Design review of the part built by this model. Coordinates are the model's own, in mm. Face numbers are marked on the shaded views. A direction names the side the tool comes from. Give positions to 0.01 mm unless a question says otherwise; leave off trailing zeros. Loops run counter-clockwise (first coordinate to the right, second up) from the corner with the lowest first, then second, coordinate; pieces in that order, holes last. Notation, with made-up numbers: M -14,76.5 L -10,76.5 A26 cw -10,110.5 Z; hole C 26.5,-10.75 d10. An arc over 180 degrees is marked long. Use CSV: the item, a comma, the result in double quotes.
from build123d import *

# Parameters (mm, degrees)
BOSS_EXTRUDE1_DEPTH = 20.32
SKETCH2_R           = 6.858
BOSS_EXTRUDE2_DEPTH = 1.27
SKETCH3_R           = 2.9845
BOSS_EXTRUDE3_DEPTH = 4.191


with BuildPart() as part:
    # Sketch1 → Boss-Extrude1 (new body)
    with BuildSketch(Plane.XY):
        Polygon((0, 0), (40.005, 0), (40.005, 27.94), (47.117, 27.94), (47.117, 31.115), (40.005, 31.115), (40.005, 40.64), (0, 40.64), (0, 31.115), (-7.112, 31.115), (-7.112, 27.94), (0, 27.94), align=None)
    extrude(amount=BOSS_EXTRUDE1_DEPTH)

    # Sketch2 → Boss-Extrude2 (add)
    with BuildSketch(Plane(origin=(0, 40.64, 0), x_dir=(1, 0, 0), z_dir=(0, 1, 0))):
        with Locations((10.886333584, -10.16)):
            Circle(SKETCH2_R)
    extrude(amount=BOSS_EXTRUDE2_DEPTH)

    # Sketch3 → Boss-Extrude3 (add)
    with BuildSketch(Plane(origin=(0, 41.91, 0), x_dir=(1, 0, 0), z_dir=(0, 1, 0))):
        with Locations((10.886333584, -10.16)):
            Circle(SKETCH3_R)
    extrude(amount=BOSS_EXTRUDE3_DEPTH)


solid = part.part
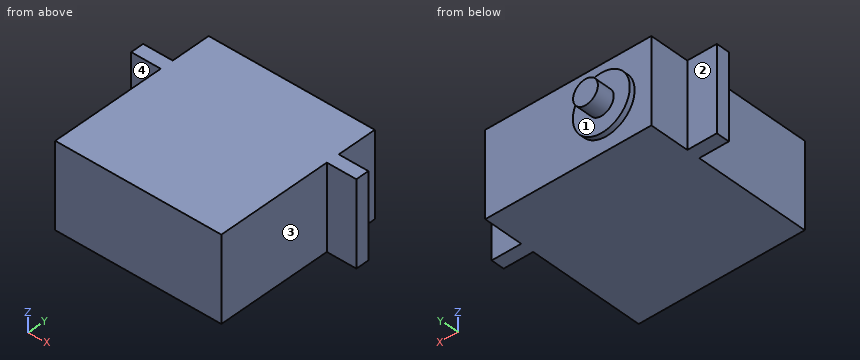
(1) We need section C-C on y = 26. State the section outline as (x, z) points (3 decimals), then the cut area to 3 significant figures.
A:
outline,"M 0,0 L 40.005,0 L 40.005,20.32 L 0,20.32 Z"
area,"813 mm²"
(2) We need section A-A on z = 10.16. State the section outline as (x, y) points (3 decimals), then the cut area to 3 significant figures.
A:
outline,"M -7.112,27.94 L 0,27.94 L 0,0 L 40.005,0 L 40.005,27.94 L 47.117,27.94 L 47.117,31.115 L 40.005,31.115 L 40.005,40.64 L 17.744,40.64 L 17.744,41.91 L 13.871,41.91 L 13.871,46.101 L 7.902,46.101 L 7.902,41.91 L 4.028,41.91 L 4.028,40.64 L 0,40.64 L 0,31.115 L -7.112,31.115 Z"
area,"1,710 mm²"
(3) We need section D-D on z = 2.5. State the section outline as (x, y) points (3 decimals), then the cut area to 3 significant figures.
A:
outline,"M -7.112,27.94 L 0,27.94 L 0,0 L 40.005,0 L 40.005,27.94 L 47.117,27.94 L 47.117,31.115 L 40.005,31.115 L 40.005,40.64 L 0,40.64 L 0,31.115 L -7.112,31.115 Z"
area,"1,670 mm²"
(4) Machinability: for the marked faces 1, 2, 3 and 4, which of the approach directions +Z, -Z, +X, -X, +Y, -Y give a long, thin tool a straight path to every point of the face, cutting with its end or side? Answer none if there is none.
A:
face 1,"+Y"
face 2,"+Z, -Z, -X, +Y"
face 3,"+Z, -Z, +X, -Y"
face 4,"+Z, -Z, -X, -Y"
(5) Wall thickness on line 1 along X through (y, z) = (19.5, 7.75) (3 decimals); line 2 along Y through (x, z) = (19.5, 9.75); line 3 along Y through (x, z) = (-4, 10) (3 decimals): over which ranges is each line inside the solid? List them lowest first. Write a range as [from, to].
A:
line 1,"[0, 40.005]"
line 2,"[0, 40.64]"
line 3,"[27.94, 31.115]"
(6) Clearance check with flat-ended pins moving along their axes: P1, Ø3.5, axis at x = -3, z = 15, coming from the -Y side; P2, Ø5, axis at x = 17.5, z = 2.5, coming from the +Y side; P3, Ø1, axis at y = 35.5, z = 13, coming from the +X side (3 decimals). State where each tip first meets the part, or that it passes through.
A:
P1,"y = 27.94"
P2,"y = 40.64"
P3,"x = 40.005"
(7) We need section B-B on x = 14.5. State the section outline as (y, z) points.
A:
outline,"M 0,0 L 40.64,0 L 40.64,4.33 L 41.91,4.33 L 41.91,15.99 L 40.64,15.99 L 40.64,20.32 L 0,20.32 Z"
